Build history of the part. All positions in model axes, mm. A direction names the side the tool comes from. Give positions to 0.01 mm unless a question says otherwise; leave off trailing zeros. Order: outer loops, then holes, each group sorted by start corner. A loop starts at its lowest first (then second) coordinate and runs counter-clockwise, first axis right, second up. Notation, with made-up numbers: (13.5, -14) - (26.5, -14) arc R25 ccw to (26.5, 10) - close; hole circle Ø1 at (54.25, 10.25). An arc over 180 degrees is marked (long way). One line per item, written item: value.
Autodesk Inventor part; units mm, degrees
ref_plane "Work Plane2" through (0, 0, -18.4174) normal (0, 0, 1) x (1, 0, 0)
ref_plane "YZ Plane" through (0, 0, 0) normal (1, 0, 0) x (0, 1, 0)
ref_plane "XZ Plane" through (0, 0, 0) normal (0, 1, 0) x (-1, 0, 0)
sketch "Sketch1" plane through (0, 0, 0) normal (0, 1, 0) x (-1, 0, 0)
  line L0 (60.406, 25.6071) -> (-60.406, 25.6071)
  line L1 (-60.406, 25.6071) -> (-60.406, -25.6071)
  line L2 (-60.406, -25.6071) -> (60.406, -25.6071)
  line L3 (60.406, -25.6071) -> (60.406, 25.6071)
  line L4 (60.406, 25.6071) -> (-60.406, -25.6071) construction
  line L5 (-60.406, 25.6071) -> (60.406, -25.6071) construction
  line L6 (-57.406, 25.6071) -> (-57.406, -25.6071)
  line L7 (57.406, -25.6071) -> (57.406, 25.6071)
  line L8 (57.406, 23.5058) -> (55.4493, 23.5058)
  line L9 (-55.4493, 23.5058) -> (-57.406, 23.5058)
  line L10 (-57.406, -33.4947) -> (-79.0126, -33.4947)
  line L11 (79.0126, -33.4947) -> (57.406, -33.4947)
  point P0 (0, 0)
  dimension "d0" = 120.812
  dimension "d1" = 51.2141
  dimension "d8" = 3
  dimension "d9" = 3
  dimension "d10" = 114.812
extrude "Extrusion1" add sketch "Sketch1" along normal blind 3
extrude "Extrusion2" add sketch "Sketch1" along normal blind 63 contours L3 L2 L7 L0 | L6 L2 L1 L0
ref_plane "Work Plane2" through (0, 0, -18.4174) normal (0, 0, 1) x (1, 0, 0)
sketch "Sketch2" plane through (0, 0, 0) normal (0, -1, 0) x (1, 0, 0)
  circle A0 centre (-50.5968, 0.5202) radius 1.75
  circle A1 centre (-28.0003, -13.4843) radius 1.75
  circle A2 centre (50.5962, 0.5202) radius 1.75
  circle A3 centre (27.9997, -13.4843) radius 1.75
  circle A4 centre (27.9997, -13.4843) radius 1.75
  circle A5 centre (50.5962, 0.5202) radius 1.75
  circle A6 centre (-28.0003, -13.4843) radius 1.75
  circle A7 centre (-50.5968, 0.5202) radius 1.75
  point P0 (0, 0)
  dimension "d12" = 3.5
  dimension "d13" = 3.5
  dimension "d14" = 3.5
  dimension "d15" = 3.5
extrude "Extrusion3" cut sketch "Sketch2" against normal up to next
sketch "Sketch4" plane through (0, 63, 0) normal (0, 1, 0) x (1, 0, 0)
  line L0 (-60.406, -8.75) -> (-56.906, -8.75)
  line L1 (-56.906, -8.75) -> (-56.906, 8.75)
  line L2 (-56.906, 8.75) -> (-60.406, 8.75)
  line L3 (-60.406, -8.75) -> (-60.406, 8.75)
  line L4 (0, 0) -> (0, 8.75)
  line L5 (60.406, -8.75) -> (56.906, -8.75)
  line L6 (56.906, -8.75) -> (56.906, 8.75)
  line L7 (56.906, 8.75) -> (60.406, 8.75)
  line L8 (60.406, -8.75) -> (60.406, 8.75)
  point P0 (-60.406, 0)
  point P1 (60.406, 0)
  dimension "d18" = 17.5
extrude "Extrusion4" cut sketch "Sketch4" against normal blind 3
sketch "Sketch6" plane through (0, 0, 0) normal (0, -1, 0) x (1, 0, 0)
  circle A0 centre (-32.4423, 8.2996) radius 1.5
  circle A1 centre (32.4417, 8.2996) radius 1.5
  point P0 (0, 0)
extrude "Extrusion5" cut sketch "Sketch6" against normal up to next
sketch "Sketch9" plane through (60.406, 0, 25.6071) normal (1, 0, 0) x (0, 0, -1)
  circle A0 centre (3, 59.0338) radius 1
  circle A1 centre (3, 38.0338) radius 1
  circle A2 centre (48.2141, 59.0338) radius 1
  circle A3 centre (48.2141, 38.0338) radius 1
  point P0 (25.6071, 0)
extrude "Extrusion7" cut sketch "Sketch9" against normal blind 200
sketch "Sketch10" plane through (0, 0, 0) normal (0, -1, 0) x (1, 0, 0)
  circle A0 centre (-28.0003, -13.4843) radius 1.75
  circle A1 centre (27.9997, -13.4843) radius 1.75
  line L0 (53.5962, 73.5112) -> (-53.5968, 73.5112)
  line L1 (-24.5003, -13.4843) -> (24.4997, -13.4843)
  line L2 (24.4997, 73.5112) -> (-24.5003, 73.5112)
  line L3 (-24.5003, -13.4843) -> (-24.5003, -2.4798)
  line L4 (-24.5003, -13.4843) -> (-13.4958, -13.4843) construction
  line L5 (-24.5003, -2.4798) -> (24.4997, -2.4798)
  line L6 (24.4997, -13.4843) -> (24.4997, -2.4798)
  point P0 (0, 0)
  dimension "d39" = 90
extrude "Extrusion8" cut sketch "Sketch10" against normal up to next contours L3 L5 L6 L1
sketch "Sketch11" plane through (0, 0, 0) normal (0, -1, 0) x (1, 0, 0)
  circle A0 centre (-38.0003, 13.0422) radius 1.75
  circle A1 centre (-14.0003, 13.0422) radius 1.75
  line L0 (-36.0003, -4.4688) -> (-36.0003, 50.5312)
  line L1 (-16.0003, 50.5312) -> (-16.0003, -4.4688)
  line L2 (-34.6078, 15.0422) -> (34.6072, 15.0422)
  point P0 (0, 0)
  dimension "d31" = 3.5
  dimension "d32" = 3.5
  dimension "d33" = 2
  dimension "d34" = 2
  dimension "d37" = 2
  dimension "d38" = 2
extrude "Extrusion9" cut sketch "Sketch11" against normal up to next
sketch "Sketch15" plane through (-60.406, 0, -25.6071) normal (-1, 0, 0) x (0, 0, 1)
  circle A0 centre (-6.7939, 16.9) radius 9.2
  point P0 (25.6071, 0)
extrude "Extrusion11" cut sketch "Sketch15" against normal through all
sketch "Sketch16" plane through (0, 0, 0) normal (0, -1, 0) x (1, 0, 0)
  line L0 (45.6757, 24.585) -> (45.6757, 11.915)
  line L1 (51.4357, 11.915) -> (51.4357, 24.585)
  line L2 (45.6757, 11.915) -> (51.4357, 11.915)
  line L3 (51.4357, 24.585) -> (45.6757, 24.585)
  line L4 (43.5557, 27) -> (53.5557, 27)
  line L5 (53.5557, 27) -> (53.5557, 9.5)
  line L6 (53.5557, 9.5) -> (43.5557, 9.5)
  line L7 (43.5557, 9.5) -> (43.5557, 27)
  line L8 (43.5557, 27) -> (53.5557, 9.5) construction
  line L9 (53.5557, 27) -> (43.5557, 9.5) construction
  point P0 (0, 0)
  point P1 (48.5557, 18.25)
  dimension "d49" = 10
  dimension "d50" = 17.5
extrude "Extrusion12" cut sketch "Sketch16" against normal up to next contours L3 L1 L2 L0 | L4 L5 L6 L7
properties part number "Kepala Tengah"
(1) Slice it at D-D, the plane z = -17.5. Give the cut face in (x, y).
Completed:
outline: (-60.41, 0) - (60.41, 0) - (60.41, 63) - (57.41, 63) - (57.41, 3) - (-57.41, 3) - (-57.41, 63) - (-60.41, 63) - close
(2) 3-axis set-ups, long thin cutter, end or side, ignore diameter. For faces 1 (the face through (53.556, 1, 18)), 2 (the face through (24.5, 1, -8)), 3 (the face through (-59, 62, 8.75)), 4 (the face through (0, 2, -25.607)), 5 (the face through (59, 63, 17)): which of +Z, -Z, +X, -X, +Y, -Y reach the whole face in a straight line?
Completed:
face 1: +Z, +Y, -Y
face 2: +Y, -Y
face 3: +X, -X, +Y
face 4: -Z, +X, -X, +Y, -Y
face 5: +Z, -Z, +X, -X, +Y
(3) Pin check, flat tips, straight feed: P1, Ø0.9, axis at x = 59, z = 3.5, coming from the +Y side; P2, Ø1.8, axis at x = -32.44, z = 8.3, coming from the +Y side (3 decimals); P3, Ø4.5, axis at x = 28, z = -13.48, coming from the +Y side. Stop position of each tip, or through.
Completed:
P1: y = 60
P2: through
P3: y = 3
(4) Slice it at A-A, the plane y = 6. Give the cut face in (x, z).
Completed:
outline: (-60.41, -25.61) - (-57.41, -25.61) - (-57.41, 25.61) - (-60.41, 25.61) - close; (57.41, -25.61) - (60.41, -25.61) - (60.41, 25.61) - (57.41, 25.61) - close
(5) Slice it at B-B, the plane x = -3.5. Give the cut face in (y, z).
Completed:
outline: (0, -25.61) - (3, -25.61) - (3, -13.48) - (0, -13.48) - close; (0, -2.48) - (3, -2.48) - (3, 25.61) - (0, 25.61) - close
(6) Slice it at C-C, the plane z = -10. Give the cut face in (x, y), and give its area (3 significant figures).
Completed:
outline: (-60.41, 0) - (-24.5, 0) - (-24.5, 3) - (-57.41, 3) - (-57.41, 63) - (-60.41, 63) - close; (24.5, 0) - (60.41, 0) - (60.41, 63) - (57.41, 63) - (57.41, 3) - (24.5, 3) - close
area: 575 mm²
(7) Pull direction X, two halves, no side cores. Call faces 6 (the face through (-60.406, 31, 0)), 7 (the face through (59, 43, -25.607)), 8 (the face through (-24.5, 1, -8)): +X half, -X half, draft (parallel to the pull), parting line (faces both ways), or undercut.
Completed:
face 6: -X half
face 7: draft
face 8: undercut
(8) Drill centre lines: line 1 (X direction, y = 34, z = -22); line 2 (Y direction, x = -12, z = 23.5). Where is each one in solid material? Low to high.
Completed:
line 1: -60.41 to -57.41, 57.41 to 60.41
line 2: 0 to 3
